Here's how the part is built. I have some questions about the finished solid (model axes, mm). Face numbers are marked on the shaded views. A direction names the side the tool comes from. Coordinates: 2 decimals unless noted, no trailing zeros. Write each loop counter-clockwise with the first axis right and the second up, starting at its lowest first coordinate (ties: lowest second). Pieces come first, ordered by that corner, then holes.
Item 1: We'd pull the mould along Y, two halves only. Please class the marked faces 1, 2 and 3: +Y half, -Y half, draft (parallel to the pull), parting line (faces both ways), or undercut.
Item 2: If we section it at D-D (z = 1.5): Please give me the cut outline in (x, y).
Item 3: For the marked faces 4 and 5, which set-ups out of +Z, -Z, +X, -X, +Y, -Y let a thin tool reach every point of the face, with its end or its side?
Item 4: I'm going to push flat-ended pins straight in: pin 1 Ø1 at (y, z) = (-34, 2) entering from -X; pin 2 Ø7.5 at (x, y) = (0, -48.42) entering from +Z (3 decimals); pin 3 Ø4 at (x, y) = (-15.5, -17) entering from -Z; pin 4 Ø1.5 at (x, z) = (-17.5, 3) entering from +Y. Where does each tip first touch, or does it pass through?
Item 5: If we section it at A-A (x = 0): Count the separate pieces of the cut face and the enclosed holes in it, then the cut area to 3 significant figures.
Item 6: If I drill on line 1 (Y direction, x = 0, z = 1.5); line 2 (Y direction, x = 0, z = 1.85); line 3 (X direction, y = -13, z = 3), over which ranges is the centre line in solid material (lowest first)?
from build123d import *

# Parameters (mm, degrees)
F0_W     = 74.6125
F0_H     = 119.0625
F0_R     = 2.38125
F0_W_2   = 33.3375
F0_H_2   = 66.675
F1_DEPTH = 6.35
F2_SIZE2 = 6.34999
F2_SIZE  = 2.53999
F3_SIZE  = 3.175


# Not quite as in the source:
# - a fillet or chamfer is up to 0.001 mm smaller than in the source, because OpenCascade refuses the exact size


with BuildPart() as f1:
    # F0 (on Top) → F1 (new body)
    with BuildSketch(Plane.XY):
        Rectangle(F0_W, F0_H)
        with Locations((0, -48.41875)):
            Circle(F0_R, mode=Mode.SUBTRACT)
        Rectangle(F0_W_2, F0_H_2, mode=Mode.SUBTRACT)
        with Locations((0, 48.41875)):
            Circle(F0_R, mode=Mode.SUBTRACT)
    extrude(amount=F1_DEPTH)

    # F2 (size 2.54 and 6.35 in the source; OpenCascade refuses exactly that, so slightly less here)
    f2_edges = [f1.edges().sort_by_distance(p)[0] for p in [
        (-16.66875, 0, 6.35),
        (0, -33.3375, 6.35),
        (16.66875, 0, 6.35),
        (0, 33.3375, 6.35),
        (0, 59.53125, 6.35),
        (37.30625, 0, 6.35),
        (0, -59.53125, 6.35),
        (-37.30625, 0, 6.35),
    ]]
    f2_side = f1.faces().sort_by_distance((0, -58.126156, 6.35))[0]
    chamfer(f2_edges, length=F2_SIZE, length2=F2_SIZE2, reference=f2_side)

    # F3
    f3_edges = [f1.edges().sort_by_distance(p)[0] for p in [
        (-2.38125, -48.41875, 6.35),
        (-2.38125, 48.41875, 6.35),
    ]]
    chamfer(f3_edges, length=F3_SIZE)


solid = f1.part
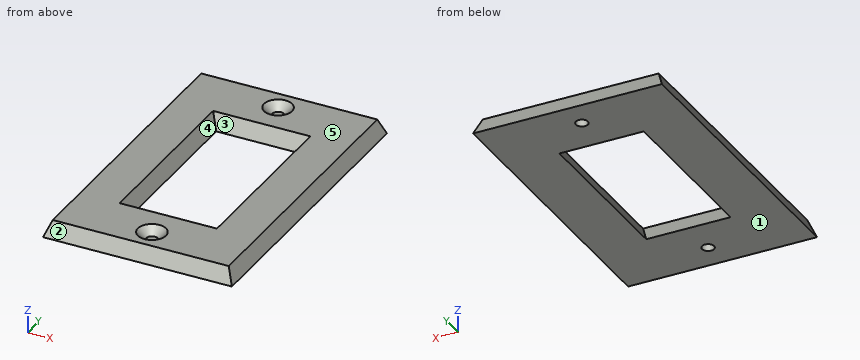
Answer list:
1. face 1: draft
1. face 2: -Y half
1. face 3: undercut
2. outline: (-36.71, -58.93) - (36.71, -58.93) - (36.71, 58.93) - (-36.71, 58.93) - close; hole (-17.27, -33.94) - (17.27, -33.94) - (17.27, 33.94) - (-17.27, 33.94) - close; hole circle Ø4.76 at (0, -48.42); hole circle Ø4.76 at (0, 48.42)
3. face 4: +Z
3. face 5: +Z, +X, -X, +Y, -Y
4. pin 1: stops at x = -36.71
4. pin 2: stops at z = 4.545
4. pin 3: stops at z = 0
4. pin 4: stops at y = 58.63
5. separate pieces: 4
5. enclosed holes: 0
5. area: 220 mm2
6. line 1: y = -58.93 to -50.8, -46.04 to -33.94, 33.94 to 46.04, 50.8 to 58.93
6. line 2: y = -58.79 to -50.8, -46.04 to -34.08, 34.08 to 46.04, 50.8 to 58.79
6. line 3: x = -36.11 to -17.87, 17.87 to 36.11
